Autodesk Inventor part; units mm, degrees
ref_plane "YZ Plane" through (0, 0, 0) normal (1, 0, 0) x (0, 1, 0)
ref_plane "XZ Plane" through (0, 0, 0) normal (0, 1, 0) x (-1, 0, 0)
ref_plane "XY Plane" through (0, 0, 0) normal (0, 0, 1) x (1, 0, 0)
sketch "スケッチ1" plane through (0, 0, 0) normal (0, 1, 0) x (-1, 0, 0)
  line L0 (0, 0) -> (0, -12.4)
  line L1 (0, -12.4) -> (5.8, -12.4)
  line L2 (5.8, -12.4) -> (5.8, -10.2)
  line L3 (5.8, -10.2) -> (7, -10.2)
  line L4 (7, -10.2) -> (7, -9.25)
  line L5 (7, -9.25) -> (5.8, -9.25)
  line L6 (5.8, -9.25) -> (5.8, -3.15)
  line L7 (5.8, -3.15) -> (7, -3.15)
  line L8 (7, -3.15) -> (7, -2.2)
  line L9 (7, -2.2) -> (5.8, -2.2)
  line L10 (5.8, -2.2) -> (5.8, 0)
  line L11 (5.8, 0) -> (0, 0)
  dimension "d1" = 12.4
  dimension "d2" = 5.8
  dimension "d3" = 0.95
  dimension "d5" = 7
  dimension "d6" = 8
extrude "押し出し1" add sketch "スケッチ1" along normal blind 7.9
sketch "スケッチ2" plane through (0, 7.9, 0) normal (0, 1, 0) x (1, 0, 0)
  line L0 (-5.8, 0) -> (0, 0)
  line L1 (0, 12.4) -> (-5.8, 12.4)
  line L2 (-5.8, 12.4) -> (-5.8, 10.2)
  line L3 (-5.8, 10.2) -> (-7, 10.2)
  line L4 (-7, 10.2) -> (-7, 9.25)
  line L5 (-7, 9.25) -> (-5.8, 9.25)
  line L6 (-5.8, 9.25) -> (-5.8, 3.15)
  line L7 (-5.8, 3.15) -> (-7, 3.15)
  line L8 (-7, 3.15) -> (-7, 2.2)
  line L9 (-7, 2.2) -> (-5.8, 2.2)
  line L10 (-5.8, 2.2) -> (-5.8, 0)
  line L11 (-5.8, 0) -> (0, 0)
  line L12 (0, 0) -> (0, 12.4)
  ellipse E0 centre (-2.9, 6.2) end of major axis (-5.8, 6.2) minor radius 6.2
  point P0 (-2.9, 0)
  point P1 (-2.9, 12.4)
  point P2 (0, 6.2)
  point P3 (-5.8, 6.2)
extrude "押し出し2" add sketch "スケッチ2" along normal blind 20 contours E0
sketch "スケッチ4" plane through (0, 0, 0) normal (0, -1, 0) x (1, 0, 0)
  line L0 (-2.2, -4.45) -> (-4.9, -4.45)
  line L1 (-4.9, -4.45) -> (-4.9, -7.95)
  line L2 (-4.9, -7.95) -> (-2.2, -7.95)
  line L3 (-2.2, -7.95) -> (-2.2, -4.45)
  line L4 (0, 0) -> (0, -12.4)
  point P0 (0, -6.2)
  point P1 (-2.2, -6.2)
  dimension "d11" = 2.7
  dimension "d12" = 3.5
  dimension "d13" = 2.2
extrude "押し出し3" add sketch "スケッチ4" along normal blind 3
properties part number "Lipo"
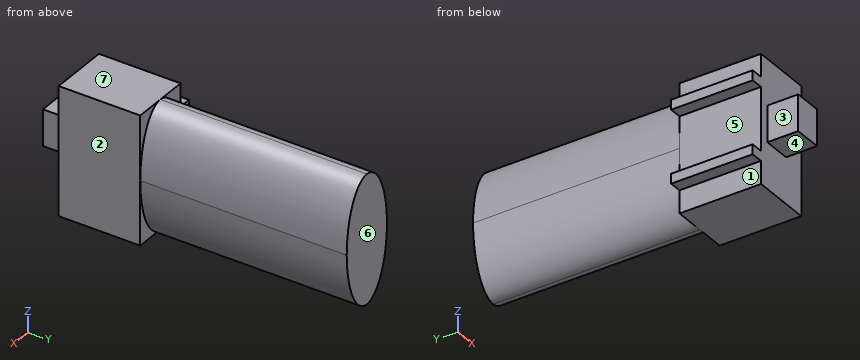
The model under review builds one solid part; all positions refer to its coordinate system, in mm. Face numbers are marked on the shaded views. A direction names the side the tool comes from. Give positions to 0.01 mm unless a question says otherwise; leave off trailing zeros. Write each loop counter-clockwise with the first axis right and the second up, starting at its lowest first coordinate (ties: lowest second). Pieces come first, ordered by that corner, then holes. Notation, with made-up numbers: M 19.25,-20.5 L 73.25,-20.5 A13 ccw 73.25,-7.5 Z; hole C -7.5,-39 d4. An arc over 180 degrees is marked long. Write item = value, one per line. Start each with the question number.
Q1. Clearance check with flat-ended pins moving along their axes: pin 1 (6 mm diameter, centred on y = 24, z = -5, fed in from +X); pin 2 (1.1 mm diameter, centred on y = 3, z = -0.5, fed in from -X); pin 3 (0.8 mm diameter, centred on x = -3, y = -1.5, fed in from -Z); pin 4 (3.5 mm diameter, centred on y = -2, z = -6.5, fed in from -X). State where each tip first meets the part, or that it passes through.
Q2. Mouldability with a two-part tool opening along Z and no side actions: class the marked faces 4, 5, 6 and 7 as released by +Z, released by -Z, zero draft, split by the parting line, or undercut.
Q3. We need section A-A (y = 7). State the section outline as (x, z) points.
Q4. Machinability: for the marked faces 1, 2 and 3, which of the approach directions +Z, -Z, +X, -X, +Y, -Y give a long, thin tool a straight path to every point of the face, cutting with its end or side? Answer none if there is none.
Q5. For line 1 (X direction, y = 2, z = -5.75); line 2 (Y direction, x = -2.25, z = -9.25); line 3 (Y direction, x = -0.75, z = -0.75), list the stretches that pass through material, from the lowest coordinate up.
Result set:
q1.pin_1 = 0
q1.pin_2 = -5.8
q1.pin_3 = -7.95
q1.pin_4 = -4.9
q2.face_4 = released by -Z
q2.face_5 = undercut
q2.face_6 = zero draft
q2.face_7 = released by +Z
q3.outline = M -7,-10.2 L -5.8,-10.2 L -5.8,-12.4 L 0,-12.4 L 0,0 L -5.8,0 L -5.8,-2.2 L -7,-2.2 L -7,-3.15 L -5.8,-3.15 L -5.8,-9.25 L -7,-9.25 Z
q4.face_1 = -Z, -X, +Y, -Y
q4.face_2 = +Z, -Z, +X, +Y, -Y
q4.face_3 = +Z, -Z, -X, -Y
q5.line_1 = -5.8 to 0
q5.line_2 = 0 to 27.9
q5.line_3 = 0 to 7.9
